from build123d import *

# Parameters (mm, degrees)
CROQUIS1_W              = 160
CROQUIS1_H              = 95
SALIENTE_EXTRUIR3_DEPTH = 5.7
REDONDEO2_R             = 1.5
CROQUIS2_R              = 2
CORTAR_EXTRUIR1_DEPTH   = 3.1


with BuildPart() as part:
    # Croquis1 → Saliente-Extruir3 (new body)
    with BuildSketch(Plane(origin=(0, 0, 0), x_dir=(1, 0, 0), z_dir=(0, 1, 0))):
        with BuildLine():
            Line((4, 120), (194, 120))
            ThreePointArc((194, 120), (196.121320344, 119.121320344), (197, 117))
            Line((197, 117), (197, 3))
            ThreePointArc((197, 3), (196.121320344, 0.878679656), (194, 0))
            Line((194, 0), (4, 0))
            ThreePointArc((4, 0), (1.878679656, 0.878679656), (1, 3))
            Line((1, 3), (1, 117))
            ThreePointArc((1, 117), (1.878679656, 119.121320344), (4, 120))
        make_face()
        with Locations((99, 60)):
            Rectangle(CROQUIS1_W, CROQUIS1_H, mode=Mode.SUBTRACT)
    extrude(amount=SALIENTE_EXTRUIR3_DEPTH)

    # Redondeo2
    redondeo2_edges = [part.edges().sort_by_distance(p)[0] for p in [
        (1.878679656, 5.7, -0.878679656),
        (99, 5.7, 0),
        (196.121320344, 5.7, -0.878679656),
        (197, 5.7, -60),
        (196.121320344, 5.7, -119.121320344),
        (99, 5.7, -120),
        (99, 5.7, -107.5),
        (19, 5.7, -60),
        (99, 5.7, -12.5),
        (179, 5.7, -60),
        (1.878679656, 5.7, -119.121320344),
        (1, 5.7, -60),
    ]]
    fillet(redondeo2_edges, radius=REDONDEO2_R)

    # Croquis2 → Cortar-Extruir1 (cut)
    with BuildSketch(Plane.XZ):
        with Locations((5, -27.38768366)):
            Circle(CROQUIS2_R)
        with Locations((5, -87.38768366)):
            Circle(CROQUIS2_R)
        with Locations((193, -27.38768366)):
            Circle(CROQUIS2_R)
        with Locations((193, -87.38768366)):
            Circle(CROQUIS2_R)
    extrude(amount=-CORTAR_EXTRUIR1_DEPTH, mode=Mode.SUBTRACT)


solid = part.part
CAD build for the part. Positions are in the model's coordinates, mm. A direction names the side the tool comes from. Round coordinates to 2 decimals unless told otherwise and drop trailing zeros. Loops run counter-clockwise (first coordinate to the right, second up) from the corner with the lowest first, then second, coordinate; pieces in that order, holes last.
(1) Wall check: line 1 along Z through (x, y) = (111, 2); line 2 along Z through (x, y) = (5, 1.1); line 3 along X through (y, z) = (1.15, -64.5). Give the ranges that are in metal, low to high.
(2) Cut at A-A (x = 145). Give the cut face in (y, z), plus the area to 3 significant figures.
(3) Two-plate mould, pull along Z, no slides. Class faces 4 (the flat face through (100, 2, 0)), 5 (the flat face through (100, 5.7, -9)), 6 (the flat face through (5, 3.1, -87)): +Z half, -Z half, draft (parallel to the pull), parting line (faces both ways), or undercut.
(4) Which spindle directions (+Z, -Z, +X, -X, +Y, -Y) get a long thin tool onto all of the face, cutting with end or side? Do faces 1 (the flat face through (98, 2, -120)), 2 (the flat face through (193, 3.1, -27)), 3 (the flat face through (179, 2, -59)). Say none if no direction does.
(5) Cut at B-B (z = -50.5). Give the cut face in (x, y).
(6) Drop flat-ended pins along their axis: pin 1 (3 mm diameter, centred on x = 5.5, z = -87, fed in from -Y); pin 2 (2 mm diameter, centred on x = 193.5, z = -87, fed in from -Y). Give the stop position or say it passes through.
Findings below:
1. line 1: z = -120 to -107.5, -12.5 to 0
1. line 2: z = -120 to -89.39, -85.39 to -29.39, -25.39 to 0
1. line 3: x = 1 to 19, 179 to 197
2. outline: (0, -120) - (4.2, -120) arc R1.5 ccw to (5.7, -118.5) - (5.7, -109) arc R1.5 ccw to (4.2, -107.5) - (0, -107.5) - close; (0, -12.5) - (4.2, -12.5) arc R1.5 ccw to (5.7, -11) - (5.7, -1.5) arc R1.5 ccw to (4.2, 0) - (0, 0) - close
2. area: 141 mm2
3. face 4: +Z half
3. face 5: draft
3. face 6: undercut
4. face 1: -Z, +X, -X, +Y, -Y
4. face 2: -Y
4. face 3: +Y, -Y
5. outline: (1, 0) - (19, 0) - (19, 4.2) arc R1.5 ccw to (17.5, 5.7) - (2.5, 5.7) arc R1.5 ccw to (1, 4.2) - close; (179, 0) - (197, 0) - (197, 4.2) arc R1.5 ccw to (195.5, 5.7) - (180.5, 5.7) arc R1.5 ccw to (179, 4.2) - close
6. pin 1: stops at y = 0
6. pin 2: stops at y = 3.1
